from build123d import *

# Parameters (mm, degrees)
BOSS_EXTRUDE1_DEPTH = 200
SKETCH2_R           = 55
BOSS_EXTRUDE2_DEPTH = 800
SKETCH4_W           = 16.611577021
SKETCH4_H           = 12.619068182
CUT_EXTRUDE1_DEPTH  = 80
ECHELLE1_SCALE      = 0.47


with BuildPart() as part:
    # Sketch1 → Boss-Extrude1 (new body)
    with BuildSketch(Plane.XY):
        with BuildLine():
            Line((-5.678147225, 60.678147225), (-37.644071104, 92.644071104))
            ThreePointArc((-37.644071104, 92.644071104), (0, 100), (37.644071104, 92.644071104))
            Line((37.644071104, 92.644071104), (5.678147225, 60.678147225))
            ThreePointArc((5.678147225, 60.678147225), (52.778396906, 30.471621661), (55.387890564, -25.421653869))
            Line((55.387890564, -25.421653869), (99.054154638, -13.721313674))
            ThreePointArc((99.054154638, -13.721313674), (86.602540378, -50), (61.410083534, -78.92275743))
            Line((61.410083534, -78.92275743), (49.709743339, -35.256493356))
            ThreePointArc((49.709743339, -35.256493356), (0, -60.943243322), (-49.709743339, -35.256493356))
            Line((-49.709743339, -35.256493356), (-61.410083534, -78.92275743))
            ThreePointArc((-61.410083534, -78.92275743), (-86.602540378, -50), (-99.054154638, -13.721313674))
            Line((-99.054154638, -13.721313674), (-55.387890564, -25.421653869))
            ThreePointArc((-55.387890564, -25.421653869), (-52.778396906, 30.471621661), (-5.678147225, 60.678147225))
        make_face()
    extrude(amount=BOSS_EXTRUDE1_DEPTH)

    # Sketch2 → Boss-Extrude2 (add)
    with BuildSketch(Plane.XY.offset(200)):
        Circle(SKETCH2_R)
    extrude(amount=-BOSS_EXTRUDE2_DEPTH)

    # Sketch4 → Cut-Extrude1 (cut)
    with BuildSketch(Plane(origin=(0, 0, -600), x_dir=(-1, 0, 0), z_dir=(0, 0, -1))):
        with Locations((3.127329512, 55.580565651)):
            Rectangle(SKETCH4_W, SKETCH4_H)
    extrude(amount=-CUT_EXTRUDE1_DEPTH, mode=Mode.SUBTRACT)


with BuildPart() as part_1:
    # Echelle1: scaled about (0.002291637, -0.041310048, -150.628565955)
    add(part.part.scale(ECHELLE1_SCALE).moved(Location((0.001214568, -0.021894325, -79.833139956))))


solid = part_1.part
Design review of the part built by this model. Coordinates are the model's own, in mm. A direction names the side the tool comes from. Round coordinates to 2 decimals unless told otherwise and drop trailing zeros. Write each loop counter-clockwise with the first axis right and the second up, starting at its lowest first coordinate (ties: lowest second). Pieces come first, ordered by that corner, then holes. Notation, with made-up numbers: (45.25, 82.5) - (73.25, 82.5) arc R28 ccw to (73.25, 116.5) - close; hole circle Ø7 at (72, -33.5). An arc over 180 degrees is marked (long way). Return JSON: item names as keys, results as strings. Group by question number.
Item 1: We need section C-C on x = 6. Write out the cut boundary in (y, z).
Item 2: We need section A-A on y = -20. Write out the cut boundary in (x, z).
Item 3: The part is to be moulded in two halves that separate along X. For faces 6 (the face through (-0.253, 46.977, -33.491)), 7 (the face through (-40.6, -23.7, -33.5)), 8 (the face through (-26.073, -26.71, -33.491)), 9 (the face through (0.384, -28.663, -33.491)), say which applies: pulls with the +X half, pulls with the -X half, needs draft (parallel to the pull), parting line crosses it, or undercut.
Item 4: Machinability: for faces 1 (the face through (26.153, -26.998, -33.491)), 2 (the face through (0, 0, -361.833)), 3 (the face through (-1, 23.135, -343)), 4 (the face through (-10.07, 35.9, -33.49)), 5 (the face through (11, 24, -79.833)), which of the approach directions +Z, -Z, +X, -X, +Y, -Y give a long, thin tool a straight path to every point of the face, cutting with its end or side? Answer none if there is none.
Item 5: Insertion check: P1, Ø4, axis at x = -10.5, y = 32.5, coming from the -Z side; P2, Ø1, axis at x = 1.5, z = -294, coming from the -Y side; P3, Ø0.8, axis at x = -2, y = 24, coming from the -Z side; P4, Ø5, axis at y = -3.5, z = -274.5, coming from the +X side. Each pin has a flat end and moves straight along its axis. Give the tip position at first contact, or say it passes through.
Item 6: For probe 1 along Z at (x, y) = (-42, -19.5); probe 2 along X at (y, z) = (-32.5, -43.5); probe 3 along Y at (x, z) = (-16.5, -97.5), list the stretches that pass through material, from the lowest coordinate up. Write a range as [from, to].
Item 7: We need section D-D on y = 9. Write out the cut boundary in (x, z).
Item 8: We need section B-B on z = -74. Write out the cut boundary in (x, y), and give its area (3 significant figures).
Model answer:
{
 "1": {"outline": "(-28.03, -79.83) - (-25.17, -79.83) - (-25.17, -361.83) - (25.12, -361.83) - (25.12, -79.83) - (27.99, -79.83) - (27.99, 14.17) - (-28.03, 14.17) - close; (31.83, -79.83) - (46.59, -79.83) - (46.59, 14.17) - (31.83, 14.17) - close"},
 "2": {"outline": "(-42.54, -79.83) - (-24.28, -79.83) - (-24.28, 14.17) - (-42.54, 14.17) - close; (-20.52, -79.83) - (-16.4, -79.83) - (-16.4, -361.83) - (16.41, -361.83) - (16.41, -79.83) - (20.53, -79.83) - (20.53, 14.17) - (-20.52, 14.17) - close; (24.28, -79.83) - (42.54, -79.83) - (42.54, 14.17) - (24.28, 14.17) - close"},
 "3": {"face 6": "parting line crosses it", "face 7": "pulls with the -X half", "face 8": "undercut", "face 9": "undercut"},
 "4": {"face 1": "+Z, -Z, -Y", "face 2": "-Z, +X, -X, +Y, -Y", "face 3": "-Z, +Y", "face 4": "+Z, -Z, -X", "face 5": "-Z"},
 "5": {"P1": "passes through", "P2": "stops at y = -25.85", "P3": "stops at z = -324.23", "P4": "stops at x = 25.83"},
 "6": {"probe 1": "z = [-79.83, 14.17]", "probe 2": "x = [-33.97, -27.62], [27.63, 33.97]", "probe 3": "y = [-19.92, 19.88]"},
 "7": {"outline": "(-27.18, -79.83) - (-24.22, -79.83) - (-24.22, -361.83) - (24.23, -361.83) - (24.23, -79.83) - (27.19, -79.83) - (27.19, 14.17) - (-27.18, 14.17) - close"},
 "8": {"outline": "(-46.55, -6.47) arc R47 ccw to (-28.86, -37.12) - (-23.36, -16.59) arc R28.64 ccw to (23.36, -16.59) - (28.86, -37.12) arc R47 ccw to (46.56, -6.47) - (26.03, -11.97) arc R28.64 ccw to (2.67, 28.5) - (17.69, 43.52) arc R47 ccw to (-17.69, 43.52) - (-2.67, 28.5) arc R28.64 ccw to (-26.03, -11.97) - close", "area": "3,740 mm²"}
}
